Could you check a few things on this drawing? It's one solid part, dimensions in mm from its lowest x, y, z. Give positions to 0.01 mm unless a question says otherwise; leave off trailing zeros. Order: outer loops, then holes, each group sorted by start corner. A loop starts at its lowest first (then second) coordinate and runs counter-clockwise, first axis right, second up.
(1) Imagine slicing it at D-D, the plane x = 62. Write out the boundary of the cut face in (y, z).
(2) If I drill on probe 1 along X at (y, z) = (15, 16); probe 2 along X at (y, z) = (26, 18); probe 3 along Z at (x, y) = (20.5, 5.5), over which ranges is the centre line in solid material (lowest first)?
(3) Imagine slicing it at C-C, the plane y = 14.5. Write out the boundary of the cut face in (x, z), then the cut area to 3 significant figures.
(4) Will these pins go through, and if not, where does the flat tip stop? pin 1 (5 mm diameter, centred on x = 70, z = 16, fed in from +Y); pin 2 (13 mm diameter, centred on x = 20, z = 16, fed in from +Y).
(5) Imagine slicing it at B-B, the plane x = 20. Write out the boundary of the cut face in (y, z), then the cut area to 3 significant figures.
(6) If we mould it in two halves opening along X, with no side actions, what happens to the marked faces 1, 2, 3 and 4? For each: released by +X, released by -X, zero draft, split by the parting line, or undercut.
(7) Imagine slicing it at A-A, the plane z = 16. Write out the boundary of the cut face in (x, y), then the cut area to 3 significant figures.
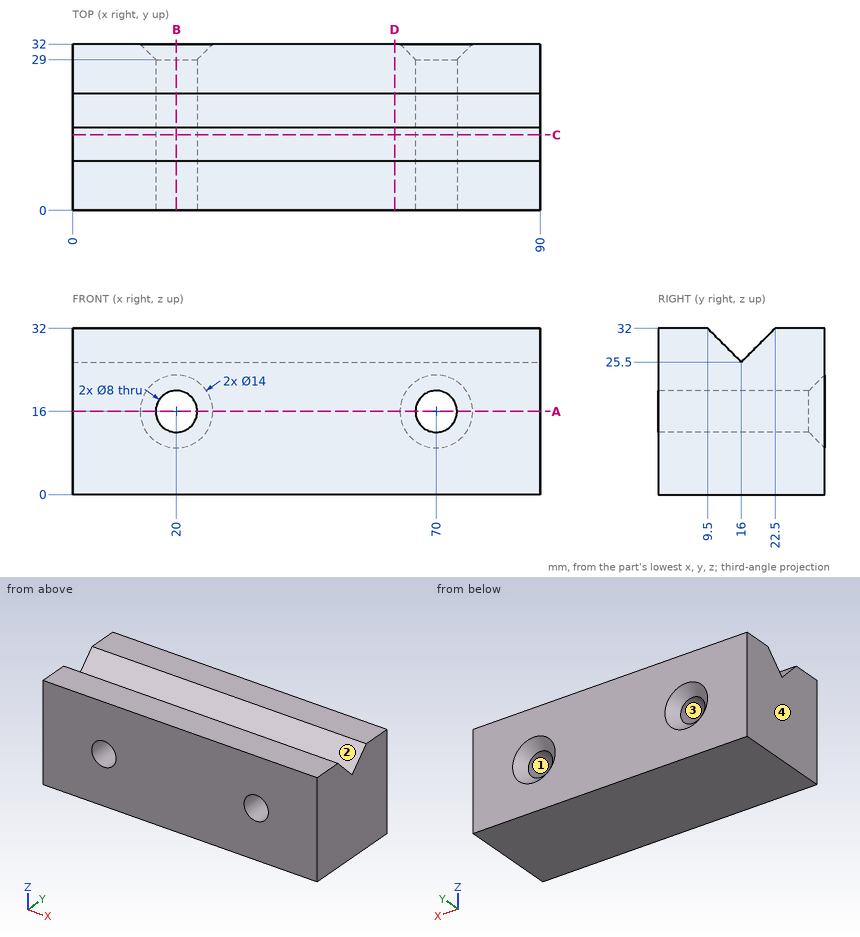
Answer block:
1. outline: (0, 0) - (32, 0) - (32, 32) - (22.5, 32) - (16, 25.5) - (9.5, 32) - (0, 32) - close
2. probe 1: x = 0 to 16, 24 to 66, 74 to 90
2. probe 2: x = 0 to 16.54, 23.46 to 66.54, 73.46 to 90
2. probe 3: z = 0 to 12.03, 19.97 to 32
3. outline: (0, 0) - (90, 0) - (90, 27) - (0, 27) - close; hole circle Ø8 at (20, 16); hole circle Ø8 at (70, 16)
3. area: 2,330 mm2
4. pin 1: passes through
4. pin 2: stops at y = 31.5
5. outline: (0, 0) - (32, 0) - (32, 9) - (29, 12) - (0, 12) - close; (0, 20) - (29, 20) - (32, 23) - (32, 32) - (22.5, 32) - (16, 25.5) - (9.5, 32) - (0, 32) - close
5. area: 717 mm2
6. face 1: undercut
6. face 2: zero draft
6. face 3: undercut
6. face 4: released by -X
7. outline: (0, 0) - (16, 0) - (16, 29) - (13, 32) - (0, 32) - close; (24, 0) - (66, 0) - (66, 29) - (63, 32) - (27, 32) - (24, 29) - close; (74, 0) - (90, 0) - (90, 32) - (77, 32) - (74, 29) - close
7. area: 2,350 mm2
